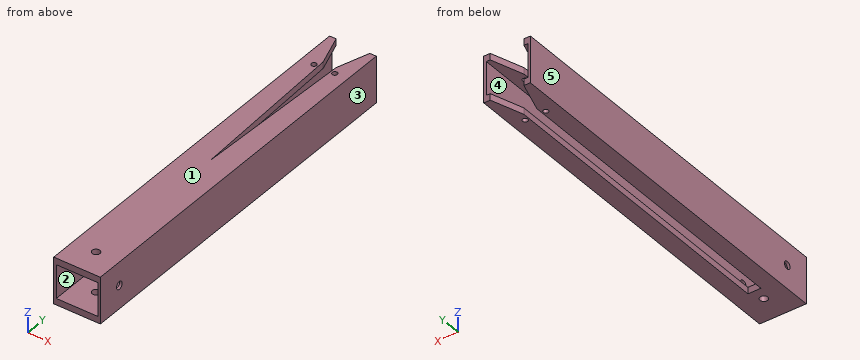
Autodesk Inventor part; units mm, degrees
ref_plane "YZ Plane" through (0, 0, 0) normal (1, 0, 0) x (0, 1, 0)
ref_plane "XZ Plane" through (0, 0, 0) normal (0, 1, 0) x (-1, 0, 0)
ref_plane "XY Plane" through (0, 0, 0) normal (0, 0, 1) x (1, 0, 0)
sketch "スケッチ1" plane through (0, 0, 0) normal (0, 1, 0) x (-1, 0, 0)
  line L0 (9, 9) -> (-9, 9)
  line L1 (-9, 9) -> (-9, -9)
  line L2 (-9, -9) -> (9, -9)
  line L3 (9, -9) -> (9, 9)
  line L4 (9, 9) -> (-9, -9) construction
  line L5 (-9, 9) -> (9, -9) construction
  point P0 (0, 0)
  dimension "d0" = 18
  dimension "d1" = 18
extrude "押し出し1" add sketch "スケッチ1" against normal blind 150
sketch "スケッチ2" plane through (0, 0, 0) normal (0, 1, 0) x (1, 0, 0)
  line L0 (-8, -6.5) -> (8, -6.5)
  line L1 (8, -6.5) -> (8, 6.5)
  line L2 (8, 6.5) -> (-8, 6.5)
  line L3 (-8, 6.5) -> (-8, -6.5)
  line L4 (-8, -6.5) -> (8, 6.5) construction
  line L5 (8, -6.5) -> (-8, 6.5) construction
  point P0 (0, 0)
  dimension "d4" = 16
  dimension "d5" = 13
extrude "押し出し2" cut sketch "スケッチ2" against normal blind 150
sketch "スケッチ4" plane through (-9, -150, 9) normal (0, 0, 1) x (1, 0, 0)
  circle A0 centre (5, 135) radius 1
  circle A1 centre (13, 135) radius 1
  point P0 (9, 150)
  dimension "d11" = 2
  dimension "d12" = 2
extrude "押し出し4" cut sketch "スケッチ4" against normal blind 150
sketch "スケッチ5" plane through (-9, -150, 9) normal (0, 0, 1) x (1, 0, 0)
  circle A0 centre (9, 15) radius 1.5
  point P0 (9, 150)
  dimension "d15" = 3
extrude "押し出し5" cut sketch "スケッチ5" against normal blind 150
sketch "スケッチ6" plane through (-9, 0, -9) normal (-1, 0, 0) x (0, 0, 1)
  circle A0 centre (9, -135) radius 1.5
  point P0 (9, 0)
  dimension "d18" = 3
extrude "押し出し6" cut sketch "スケッチ6" against normal blind 150
thread "ねじ1"
thread "ねじ2"
sketch "スケッチ7" plane through (-9, 0, 9) normal (0, 0, 1) x (1, 0, 0)
  line L0 (9, 0) -> (9, -75)
  line L1 (9, 0) -> (6, 0)
  line L2 (0, 0) -> (18, 0)
  line L3 (6, 0) -> (9, -75)
  line L4 (9, 0) -> (12, 0)
  line L5 (12, 0) -> (9, -75)
  point P0 (12, 0)
  dimension "d25" = 75
  dimension "d26" = 3
  dimension "d27" = 3
extrude "押し出し7" cut sketch "スケッチ7" against normal blind 30
sketch "スケッチ8" plane through (-9, -150, 9) normal (0, 0, 1) x (1, 0, 0)
  line L0 (9, 150) -> (15.5, 150)
  line L1 (18, 150) -> (12, 150)
  line L2 (9, 150) -> (9, 130)
  line L3 (9, 130) -> (15.5, 150)
  line L4 (9, 150) -> (2.5, 150)
  line L5 (2.5, 150) -> (9, 130)
  dimension "d30" = 6.5
  dimension "d31" = 20
  dimension "d32" = 6.5
extrude "押し出し8" cut sketch "スケッチ8" against normal blind 30
sketch "スケッチ9" plane through (9, -150, -9) normal (0, 0, -1) x (-1, 0, 0)
  line L0 (9, 150) -> (9, 20)
  line L1 (11.5088, 137.7193) -> (9, 75)
  line L2 (11.5088, 137.7193) -> (11.5088, 20)
  line L3 (11.5088, 20) -> (9, 20)
  line L4 (2.5, 150) -> (6.4912, 137.7193)
  line L5 (6.4912, 137.7193) -> (6.4912, 20)
  line L6 (6.4912, 20) -> (9, 20)
  line L7 (6.4912, 137.7193) -> (11.5088, 137.7193)
  dimension "d35" = 130
extrude "押し出し9" cut sketch "スケッチ9" against normal blind 10
sketch "スケッチ10" plane through (0, -150, 0) normal (0, -1, 0) x (1, 0, 0)
  line L0 (-9, -9) -> (-9, 9)
  line L1 (9, 9) -> (-9, 9)
  line L2 (-9, 9) -> (-9, -9)
  line L3 (-9, -9) -> (9, -9)
  line L4 (9, -9) -> (9, 9)
  line L5 (9, 9) -> (-9, -9) construction
  line L6 (-9, 9) -> (9, -9) construction
  point P0 (0, 0)
extrude "押し出し10" cut sketch "スケッチ10" against normal blind 5
properties part number "square_bar" material "アルミニウム 6061"
Input: part model. Units: mm. Frame: model coordinates. Face numbers are marked on the shaded views. A direction names the side the tool comes from. Coordinates: 2 decimals unless noted, no trailing zeros. Write each loop counter-clockwise with the first axis right and the second up, starting at its lowest first coordinate (ties: lowest second). Pieces come first, ordered by that corner, then holes. Notation, with made-up numbers: (24, 60.25) -> (78, 60.25) arc R22 cw to (78, 92.25) -> close; hole circle Ø6 at (65.5, 12.25). An arc over 180 degrees is marked (long way). Answer as a JSON object with one key per item and string values.
1. Material intervals for line 1 (Y direction, x = 0, z = -7.3); line 2 (Z direction, x = -8.45, y = -135); line 3 (Z direction, x = -6, y = -53), sorted ascending. Write a range as from..to.
Result set:
{"line 1": "y = -145..-136.5, -133.5..-130", "line 2": "z = -9..-1.5, 1.5..9", "line 3": "z = -9..-6.5, 6.5..9"}
2. Section A-A on z = 4. Return the cut outline in (x, y).
Result set:
{"outline": "(-9, -145) -> (-8, -145) -> (-8, 0) -> (-9, 0) -> close; (8, -145) -> (9, -145) -> (9, 0) -> (8, 0) -> close"}
3. Access query for the marked faces 4 and 5. Directions: +Z, -Z, +X, -X, +Y, -Y. A direction counts if a zero-diameter tool reaches every point of the face in a straight line with its end or side. Return the directions, or none.
Result set:
{"face 4": "+Y, -Y", "face 5": "+Z, -Z, -X, +Y, -Y"}
4. Section B-B on y = -67.5. Return the cut outline in (x, z).
Result set:
{"outline": "(-9, -9) -> (-2.51, -9) -> (-2.51, -6.5) -> (-8, -6.5) -> (-8, 6.5) -> (-0.3, 6.5) -> (-0.3, 9) -> (-9, 9) -> close; (0.3, 6.5) -> (8, 6.5) -> (8, -6.5) -> (2.51, -6.5) -> (2.51, -9) -> (9, -9) -> (9, 9) -> (0.3, 9) -> close"}
5. Section C-C on y = -91. Return the cut outline in (x, z).
Result set:
{"outline": "(-9, -9) -> (-2.51, -9) -> (-2.51, -6.5) -> (-8, -6.5) -> (-8, 6.5) -> (8, 6.5) -> (8, -6.5) -> (2.51, -6.5) -> (2.51, -9) -> (9, -9) -> (9, 9) -> (-9, 9) -> close"}
6. First-contact query: P1, Ø1.8, axis at x = 0, y = -135, coming from the +Z side; P2, Ø2, axis at x = -1, z = -8.5, coming from the +Y side. Flat tips, straight axial feed; report the tip coordinate or a pass-through.
Result set:
{"P1": "passes through", "P2": "stops at y = -130"}
7. Mould query, pull axis Z, two halves, no side actions, for the marked faces 1, 2 and 3. Classes: released by +Z, released by -Z, zero draft, split by the parting line, or undercut.
Result set:
{"face 1": "released by +Z", "face 2": "undercut", "face 3": "zero draft"}
